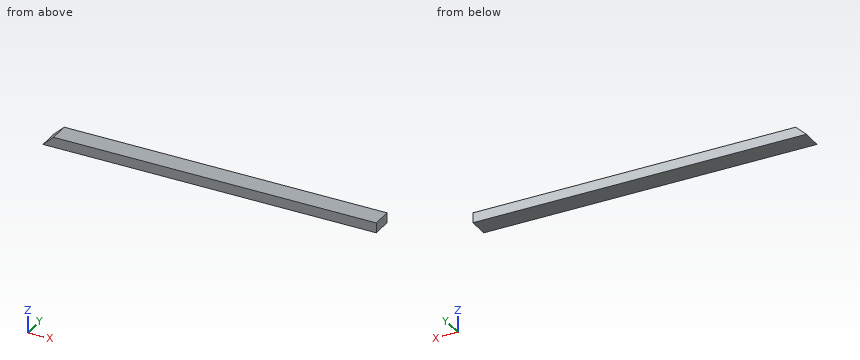
Autodesk Inventor part; units mm, degrees
ref_plane "YZ Plane" through (0, 0, 0) normal (1, 0, 0) x (0, 1, 0)
ref_plane "XZ Plane" through (0, 0, 0) normal (0, 1, 0) x (-1, 0, 0)
ref_plane "XY Plane" through (0, 0, 0) normal (0, 0, 1) x (1, 0, 0)
ref_plane "Work Plane1" through (0, 0, 0) normal (0, 0, 1) x (1, 0, 0)
sketch "Sketch1" plane through (0, 0, 0) normal (0, 0, 1) x (1, 0, 0)
  line L0 (-55.6518, 0) -> (0, 0)
  line L1 (-55.6518, 0) -> (-55.6518, -101.6)
  line L2 (0, -101.6) -> (-55.6518, -101.6)
  line L3 (0, 0) -> (0, -101.6)
  line L4 (1549.4, -50.8) -> (1651, -50.8)
  line L5 (1651, -50.8) -> (1651, 0)
  line L6 (1549.4, 0) -> (1651, 0)
  line L7 (1549.4, -50.8) -> (1549.4, 0)
  line L8 (-55.6518, -101.6) -> (1600.2, -101.6)
  line L9 (1600.2, -101.6) -> (1600.2, 0)
  line L10 (1600.2, 0) -> (-55.6518, 0)
  line L11 (-55.6518, 0) -> (-55.6518, -101.6)
  point P0 (0, 0)
extrude "Extrusion1" add sketch "Sketch1" along normal blind 50.8 contours L0 L3 L2 L1 | L10 L7 L4 L9 L8 L3 | L6 L9 L4 L7
sketch "Sketch3" plane through (-55.6518, -101.6, 0) normal (0, -1, 0) x (1, 0, 0)
  line L0 (0, 0) -> (101.6, 0)
  line L1 (101.6, 0) -> (1270, 1117.6)
  line L2 (1270, 1117.6) -> (1270, 1219.2)
  line L3 (1270, 1219.2) -> (0, 0)
  line L4 (0, 0) -> (101.6, 0)
  line L5 (101.6, 0) -> (1270, 1117.6)
  line L6 (1270, 1117.6) -> (1270, 1219.2)
  line L7 (1270, 1219.2) -> (0, 0)
  line L8 (0, 0) -> (0, 50.8)
  line L9 (0, 0) -> (0, 50.8)
  line L10 (0, 50.8) -> (52.9167, 50.8)
  line L11 (0, 50.8) -> (1655.8518, 50.8)
  line L12 (0, 0) -> (1655.8518, 0)
  line L13 (52.9167, 50.8) -> (0, 0)
  point P0 (55.6518, 0)
  point P1 (52.9167, 50.8)
extrude "Extrusion3" cut sketch "Sketch3" against normal blind 101.6 contours L8 L10 L3
ref_plane "Work Plane2" through (1620.7482, -50.8, -965.2) normal (0, 1, 0) x (0, 0, -1)
sketch "Sketch4" plane through (1600.2, 0, 50.8) normal (0, 1, 0) x (1, 0, 0)
  line L0 (-30.2518, 1981.2) -> (-30.2518, 50.8)
  line L1 (-30.2518, 50.8) -> (71.3482, 50.8)
  line L2 (71.3482, 50.8) -> (71.3482, 1981.2)
  line L3 (71.3482, 1981.2) -> (-30.2518, 1981.2)
  line L4 (-30.2518, 1981.2) -> (-30.2518, 50.8)
  line L5 (-30.2518, 50.8) -> (71.3482, 50.8)
  line L6 (71.3482, 50.8) -> (71.3482, 1981.2)
  line L7 (71.3482, 1981.2) -> (-30.2518, 1981.2)
  line L8 (20.5482, 50.8) -> (0, 50.8)
  line L9 (-1602.9352, 0) -> (0, 0)
  line L10 (0, 50.8) -> (0, 0)
  line L11 (0, 0) -> (20.5482, 0)
  line L12 (20.5482, 0) -> (20.5482, 50.8)
  point P0 (-1600.2, 50.8)
  point P1 (20.5482, 50.8)
extrude "Extrusion4" add sketch "Sketch4" against normal blind 101.6 contours L1 L12 L11 L10
properties part number "2X4X65.191" material "Wood (Birch)"
Could you check a few things on this model? Use its own coordinates, in mm. Give positions to 0.01 mm unless a question says otherwise; leave off trailing zeros. Order: outer loops, then holes, each group sorted by start corner. A loop starts at its lowest first (then second) coordinate and runs counter-clockwise, first axis right, second up. Notation, with made-up numbers: (-25, 60) - (-14, 60) arc R14 cw to (-14, 85) - close; hole circle Ø4 at (27, -0.5). An arc over 180 degrees is marked (long way). One line per question, with ' | ' between items. Start each with the question number.
Item 1: I need wall thicknesses on probe 1 along X at (y, z) = (-85.5, 9); probe 2 along X at (y, z) = (-52.5, 11). Which ranges of each line are inside material? Lowest first, please. Write a range as [from, to].
Item 2: I want a section at A-A on y = -73.5. Write out the boundary of the cut face in (x, z).
Item 3: I'm going to push a flat-ended pin straight in: pin 1 Ø10 at (y, z) = (-70.5, 42) entering from -X. Where does the tip first touch, or does it pass through?
Item 4: I want a section at B-B on z = 40. Write out the boundary of the cut face in (x, y), then the cut area to 3 significant figures.
Verdict:
1) probe 1: [-46.28, 1620.75] | probe 2: [-44.19, 1620.75]
2) outline: (-55.65, 0) - (1620.75, 0) - (1620.75, 50.8) - (-2.74, 50.8) - close
3) pin 1: x = -17.11
4) outline: (-13.99, -101.6) - (1620.75, -101.6) - (1620.75, 0) - (-13.99, 0) - close | area: 166,000 mm^2
